```python
from build123d import *

# Parameters (mm, degrees)
F1_DEPTH  = 25
F2_W      = 90
F2_H      = 10
F2_W_2    = 70
F3_DEPTH  = 40
F4_R      = 15
F5_DEPTH  = 25
F6_SIZE   = 2
F8_D      = 25
F10_DEPTH = 25


with BuildPart() as f1:
    # F0 (on Front) → F1 (new body, symmetric)
    with BuildSketch(Plane.XZ):
        Polygon((-250, 0), (0, 0), (0, 10), (-200, 10), (-200, 50), (-250, 50), align=None)
    extrude(amount=F1_DEPTH, both=True)

    # F2 (on face) → F3 (join)
    with BuildSketch(Plane.XY.offset(10)):
        with Locations((-155, 20)):
            Rectangle(F2_W, F2_H)
        with Locations((-35, -20)):
            Rectangle(F2_W_2, F2_H)
    extrude(amount=F3_DEPTH)

    # F4 (on face) → F5 (join)
    with BuildSketch(Plane(origin=(-250, 0, 0), x_dir=(0, -1, 0), z_dir=(-1, 0, 0))):
        with Locations((0, 25)):
            Circle(F4_R)
    extrude(amount=F5_DEPTH)

    # F6
    f6_edges = [f1.edges().sort_by_distance(p)[0] for p in [
        (-275, 15, 25),
    ]]
    chamfer(f6_edges, length=F6_SIZE)

    # F8 (through all)
    with Locations(Plane.XY.offset(50)):
        with Locations((-225, 0)):
            Hole(F8_D / 2)

    # F9 (on face) → F10 (cut, through all)
    with BuildSketch(Plane(origin=(-275, 0, 0), x_dir=(0, -1, 0), z_dir=(-1, 0, 0))):
        with BuildLine():
            Line((5, 42), (-5, 42))
            Line((-5, 42), (-5, 37))
            ThreePointArc((-5, 37), (0, 38), (5, 37))
            Line((5, 37), (5, 42))
        make_face()
        with BuildLine():
            ThreePointArc((5, 37), (0, 38), (-5, 37))
            Line((-5, 37), (-5, 35))
            Line((-5, 35), (5, 35))
            Line((5, 35), (5, 37))
        make_face()
    extrude(amount=-F10_DEPTH, mode=Mode.SUBTRACT)


solid = f1.part
```
Geometry check sheet. Reference: the model listing, model coordinates, mm. A direction names the side the tool comes from. Coordinates: 2 decimals unless noted, no trailing zeros. Write each loop counter-clockwise with the first axis right and the second up, starting at its lowest first coordinate (ties: lowest second). Pieces come first, ordered by that corner, then holes. Notation, with made-up numbers: M 30.5,25.5 L 43.5,25.5 A29 ccw 43.5,52.5 Z; hole C 44.5,64 d1. An arc over 180 degrees is marked long. Answer as a JSON object with one key per item and string values.
1. Section check A-A, the plane z = 25. Enter the section's corners in (x, y), plus the area to 3 significant figures.
Answers below:
{"outline": "M -275,-13 L -273,-15 L -250,-15 L -250,-25 L -200,-25 L -200,15 L -110,15 L -110,25 L -250,25 L -250,15 L -273,15 L -275,13 Z; M -70,-25 L 0,-25 L 0,-15 L -70,-15 Z; hole C -225,0 d25", "area": "4,360 mm²"}
2. Go/stop test with flat-tipped pins: pin 1 Ø5 at (y, z) = (5, 9.5) entering from -X; pin 2 Ø2 at (x, z) = (-262.5, 36) entering from -Y; pin 3 Ø2 at (x, y) = (-63, 4) entering from +Z. Record where each tip stops, or that it passes through.
Answers below:
{"pin 1": "stops at x = -274.21", "pin 2": "stops at y = -11.18", "pin 3": "stops at z = 10"}
3. Section check D-D, the plane y = -18.5. Enter the section's corners in (x, z).
Answers below:
{"outline": "M -250,0 L 0,0 L 0,50 L -70,50 L -70,10 L -200,10 L -200,50 L -250,50 Z"}
4. Scan lines: L1, parallel to X at y = -18.5, z = 40.5; L2, parallel to Y at x = -225, z = 10.5; L3, parallel to Y at x = -116.5, z = 44. Record each from-to range of solid material in increasing order.
Answers below:
{"L1": "x = -250 to -200, -70 to 0", "L2": "y = -25 to -12.5, 12.5 to 25", "L3": "y = 15 to 25"}
5. Section check B-B, the plane y = 0. Enter the section's corners in (x, z), plus the area to 3 significant figures.
Answers below:
{"outline": "M -275,12 L -273,10 L -250,10 L -250,0 L -237.5,0 L -237.5,50 L -250,50 L -250,35 L -275,35 Z; M -212.5,0 L 0,0 L 0,10 L -200,10 L -200,50 L -212.5,50 Z", "area": "3,870 mm²"}
6. Tool access check on faces 1 (the cylindrical face through (-261.34, 0.59, 10.01)), 2 (the flat face through (-35, -15, 30)), 3 (the flat face through (-263, 0, 35)), 4 (the flat face through (-110, 20, 30)), 5 (the flat face through (-156, 15, 30)). Record the directions out of +Z, -Z, +X, -X, +Y, -Y that give a thin tool (end or side, any length) a straight path to the whole face; none if there is none.
Answers below:
{"face 1": "-X", "face 2": "+Z, +X, +Y", "face 3": "+Z, -X", "face 4": "+Z, +X, +Y, -Y", "face 5": "+Z, +X, -Y"}
7. Draft check along X on faces 6 (the flat face through (-200, -5, 30)), 7 (the flat face through (-275, 0, 25)), 8 (the flat face through (-127, -25, 9)). Enter one of: released by +X, released by -X, zero draft, split by the parting line, or undercut.
Answers below:
{"face 6": "undercut", "face 7": "released by -X", "face 8": "zero draft"}
8. Section check C-C, the plane x = -225. Enter the section's corners in (y, z).
Answers below:
{"outline": "M -25,0 L -12.5,0 L -12.5,50 L -25,50 Z; M 12.5,0 L 25,0 L 25,50 L 12.5,50 Z"}
